Model file for the job. Use its own axes, mm. A direction names the side the tool comes from. Round coordinates to 2 decimals unless told otherwise and drop trailing zeros. Order: outer loops, then holes, each group sorted by start corner. A loop starts at its lowest first (then second) coordinate and runs counter-clockwise, first axis right, second up. Notation, with made-up numbers: (-7.75, 30) -> (24.25, 30) arc R15 ccw to (24.25, 41) -> close; hole circle Ø6 at (42.5, 12.5). An arc over 180 degrees is marked (long way). Use CSV: the item, a comma, the result in double quotes.
```python
from build123d import *

# Parameters (mm, degrees)
SKETCH_W     = 173
SKETCH_H     = 318
PAD_DEPTH    = 10
SKETCH001_W  = 131
SKETCH001_H  = 145
PAD001_DEPTH = 5
SKETCH002_R  = 3
POCKET_DEPTH = 5


with BuildPart() as part:
    # Sketch → Pad (new body)
    with BuildSketch(Plane.XZ):
        Rectangle(SKETCH_W, SKETCH_H)
    extrude(amount=-PAD_DEPTH)

    # Sketch001 → Pad001 (join)
    with BuildSketch(Plane.XZ):
        with Locations((0, 86.5)):
            Rectangle(SKETCH001_W, SKETCH001_H)
    extrude(amount=PAD001_DEPTH)

    # Sketch002 → Pocket (cut)
    with BuildSketch(Plane.XZ):
        with Locations((-52.5, 150)):
            Circle(SKETCH002_R)
        with Locations((-52.5, 84)):
            Circle(SKETCH002_R)
        with Locations((-52.5, 24)):
            Circle(SKETCH002_R)
        with Locations((55.5, 150)):
            Circle(SKETCH002_R)
        with Locations((55.5, 84)):
            Circle(SKETCH002_R)
        with Locations((55.5, 24)):
            Circle(SKETCH002_R)
        with BuildLine():
            ThreePointArc((3, 104), (0, 107), (-3, 104))
            Line((-3, 104), (-3, 96))
            ThreePointArc((-3, 96), (0, 87), (3, 96))
            Line((3, 104), (3, 96))
        make_face()
    extrude(amount=POCKET_DEPTH, mode=Mode.SUBTRACT)


solid = part.part
```
Q1. Mould opens along Z. For faces 3 (the flat face through (-86.5, 5, -2)), 4 (the flat face through (55, 0, 84)), 5 (the flat face through (-1, 5, -159)) say: +Z half, -Z half, draft (parallel to the pull), parting line (faces both ways), or undercut.
From the geometry:
face 3,"draft"
face 4,"undercut"
face 5,"-Z half"
Q2. Which spindle directions (+Z, -Z, +X, -X, +Y, -Y) get a long thin tool onto all of the face, cutting with end or side? Do faces 1 (the flat face through (86.5, 5, -2)), 2 (the cylindrical face through (53.1, -2.5, 82.2)). Say none if no direction does.
From the geometry:
face 1,"+Z, -Z, +X, +Y, -Y"
face 2,"-Y"
Q3. Cut at A-A (z = 24). Give the cut face in (x, y).
From the geometry:
outline,"(-86.5, 0) -> (-65.5, 0) -> (-65.5, -5) -> (-55.5, -5) -> (-55.5, 0) -> (-49.5, 0) -> (-49.5, -5) -> (52.5, -5) -> (52.5, 0) -> (58.5, 0) -> (58.5, -5) -> (65.5, -5) -> (65.5, 0) -> (86.5, 0) -> (86.5, 10) -> (-86.5, 10) -> close"
Q4. Probe line 1 along Z through (x, y) = (55.5, -2.4); line 2 along X through (y, z) = (-2.15, 150); line 3 along Y through (x, z) = (41, 2). List the from-to ranges inside material, lowest first.
From the geometry:
line 1,"z = 14 to 21, 27 to 81, 87 to 147, 153 to 159"
line 2,"x = -65.5 to -55.5, -49.5 to 52.5, 58.5 to 65.5"
line 3,"y = 0 to 10"
Q5. Cut at D-D (z = 92). Give the cut face in (x, y).
From the geometry:
outline,"(-86.5, 0) -> (-65.5, 0) -> (-65.5, -5) -> (-5, -5) -> (-5, 0) -> (5, 0) -> (5, -5) -> (65.5, -5) -> (65.5, 0) -> (86.5, 0) -> (86.5, 10) -> (-86.5, 10) -> close"
Q6. Cut at B-B (x = -45.5). Give the cut face in (y, z), plus the area to 4 significant figures.
From the geometry:
outline,"(-5, 14) -> (0, 14) -> (0, -159) -> (10, -159) -> (10, 159) -> (-5, 159) -> close"
area,"3,905 mm²"
Q7. Cut at C-C (x = 55.5). Give the cut face in (y, z), plus the area to 4 significant figures.
From the geometry:
outline,"(-5, 14) -> (0, 14) -> (0, -159) -> (10, -159) -> (10, 159) -> (-5, 159) -> (-5, 153) -> (0, 153) -> (0, 147) -> (-5, 147) -> (-5, 87) -> (0, 87) -> (0, 81) -> (-5, 81) -> (-5, 27) -> (0, 27) -> (0, 21) -> (-5, 21) -> close"
area,"3,815 mm²"
Q8. Pin check, flat tips, straight feed: pin 1 (5.5 mm diameter, centred on y = -2.5, z = 99, fed in from +X); pin 2 (1.5 mm diameter, centred on y = -1.5, z = 55.5, fed in from -X); pin 3 (9 mm diameter, centred on x = 0, z = 92, fed in from -Y). Stop position of each tip, or through.
From the geometry:
pin 1,"stops at x = 86.5"
pin 2,"stops at x = -65.5"
pin 3,"stops at y = 0"
